from build123d import *

# Parameters (mm, degrees)
F1_DEPTH = 101.6
F3_DEPTH = 6.35
F4_R     = 3.175
F5_DEPTH = 50.801
F6_R     = 6.35
F7_DEPTH = 6.35


with BuildPart() as f1:
    # F0 (on Front) → F1 (new body)
    with BuildSketch(Plane.XZ):
        Polygon((0, 50.8), (0, 0), (148.59, 0), (148.59, 12.7), (135.89, 12.7), (135.89, 25.4), (123.19, 25.4), (123.19, 38.1), (110.49, 38.1), (110.49, 50.8), align=None)
    extrude(amount=F1_DEPTH)

    # F2 (on face) → F3 (cut)
    with BuildSketch(Plane.XY.offset(50.8)):
        with BuildLine():
            ThreePointArc((25.4, -31.75), (29.890128, -29.890128), (31.75, -25.4))
            ThreePointArc((31.75, -25.4), (29.890128, -20.909872), (25.4, -19.05))
            ThreePointArc((25.4, -19.05), (19.05, -25.4), (25.4, -31.75))
        make_face()
        with BuildLine():
            ThreePointArc((25.4, -19.05), (29.890128, -20.909872), (31.75, -25.4))
            ThreePointArc((31.75, -25.4), (29.890128, -29.890128), (25.4, -31.75))
            Line((25.4, -31.75), (101.6, -31.75))
            ThreePointArc((101.6, -31.75), (95.25, -25.4), (101.6, -19.05))
            Line((101.6, -19.05), (25.4, -19.05))
        make_face()
        with BuildLine():
            ThreePointArc((107.95, -25.4), (106.090128, -20.909872), (101.6, -19.05))
            ThreePointArc((101.6, -19.05), (95.25, -25.4), (101.6, -31.75))
            ThreePointArc((101.6, -31.75), (106.090128, -29.890128), (107.95, -25.4))
        make_face()
        with BuildLine():
            ThreePointArc((31.75, -76.2), (29.890128, -80.690128), (25.4, -82.55))
            Line((25.4, -82.55), (101.6, -82.55))
            ThreePointArc((101.6, -82.55), (95.25, -76.2), (101.6, -69.85))
            Line((101.6, -69.85), (25.4, -69.85))
            ThreePointArc((25.4, -69.85), (29.890128, -71.709872), (31.75, -76.2))
        make_face()
        with BuildLine():
            ThreePointArc((25.4, -69.85), (19.05, -76.2), (25.4, -82.55))
            ThreePointArc((25.4, -82.55), (29.890128, -80.690128), (31.75, -76.2))
            ThreePointArc((31.75, -76.2), (29.890128, -71.709872), (25.4, -69.85))
        make_face()
        with BuildLine():
            ThreePointArc((101.6, -69.85), (95.25, -76.2), (101.6, -82.55))
            ThreePointArc((101.6, -82.55), (106.090128, -80.690128), (107.95, -76.2))
            ThreePointArc((107.95, -76.2), (106.090128, -71.709872), (101.6, -69.85))
        make_face()
    extrude(amount=-F3_DEPTH, mode=Mode.SUBTRACT)

    # F4 (on face) → F5 (cut, through all)
    with BuildSketch(Plane.XY.offset(50.8)):
        with Locations((101.6, -50.8)):
            Circle(F4_R)
        with Locations((63.5, -50.8)):
            Circle(F4_R)
        with BuildLine():
            ThreePointArc((25.4, -28.575), (27.645064, -27.645064), (28.575, -25.4))
            ThreePointArc((28.575, -25.4), (27.645064, -23.154936), (25.4, -22.225))
            ThreePointArc((25.4, -22.225), (22.225, -25.4), (25.4, -28.575))
        make_face()
        with BuildLine():
            ThreePointArc((25.4, -22.225), (27.645064, -23.154936), (28.575, -25.4))
            ThreePointArc((28.575, -25.4), (27.645064, -27.645064), (25.4, -28.575))
            Line((25.4, -28.575), (101.6, -28.575))
            ThreePointArc((101.6, -28.575), (98.425, -25.4), (101.6, -22.225))
            Line((101.6, -22.225), (25.4, -22.225))
        make_face()
        with BuildLine():
            ThreePointArc((104.775, -25.4), (103.845064, -23.154936), (101.6, -22.225))
            ThreePointArc((101.6, -22.225), (98.425, -25.4), (101.6, -28.575))
            ThreePointArc((101.6, -28.575), (103.845064, -27.645064), (104.775, -25.4))
        make_face()
        with Locations((25.4, -50.8)):
            Circle(F4_R)
        with BuildLine():
            ThreePointArc((25.4, -79.375), (27.645064, -78.445064), (28.575, -76.2))
            ThreePointArc((28.575, -76.2), (27.645064, -73.954936), (25.4, -73.025))
            ThreePointArc((25.4, -73.025), (22.225, -76.2), (25.4, -79.375))
        make_face()
        with BuildLine():
            ThreePointArc((25.4, -73.025), (27.645064, -73.954936), (28.575, -76.2))
            ThreePointArc((28.575, -76.2), (27.645064, -78.445064), (25.4, -79.375))
            Line((25.4, -79.375), (101.6, -79.375))
            ThreePointArc((101.6, -79.375), (98.425, -76.2), (101.6, -73.025))
            Line((101.6, -73.025), (25.4, -73.025))
        make_face()
        with BuildLine():
            ThreePointArc((104.775, -76.2), (103.845064, -73.954936), (101.6, -73.025))
            ThreePointArc((101.6, -73.025), (98.425, -76.2), (101.6, -79.375))
            ThreePointArc((101.6, -79.375), (103.845064, -78.445064), (104.775, -76.2))
        make_face()
    extrude(amount=-F5_DEPTH, mode=Mode.SUBTRACT)

    # F6 (on face) → F7 (cut)
    with BuildSketch(Plane.XY.offset(50.8)):
        with Locations((101.6, -50.8)):
            Circle(F6_R)
        with Locations((63.5, -50.8)):
            Circle(F6_R)
        with Locations((25.4, -50.8)):
            Circle(F6_R)
    extrude(amount=-F7_DEPTH, mode=Mode.SUBTRACT)


solid = f1.part
Can you work these out from the model? Positions are in its coordinate system, mm. A direction names the side the tool comes from. Round coordinates to 2 decimals unless told otherwise and drop trailing zeros. Loops run counter-clockwise (first coordinate to the right, second up) from the corner with the lowest first, then second, coordinate; pieces in that order, holes last. Notation, with made-up numbers: (-0.75, -5) - (15.25, -5) arc R13 cw to (15.25, 19) - close; hole circle Ø5 at (16, 12). An arc over 180 degrees is marked (long way). Write item = value, one per line. Start each with the question number.
(1) If we section it at C-C (y = -10.5): Please give me the cut outline in (x, z), and give its area (3 significant figures).
(2) For faces 1 (the face through (22.226, -25.33, 22.536)), 2 (the face through (66, -54, 44.45)), 3 (the face through (56, -50, 50.8)), which set-ups out of +Z, -Z, +X, -X, +Y, -Y let a thin tool reach every point of the face, with its end or its side?
(3) If we section it at A-A (x = 63.5): Please give me the cut outline in (y, z) (3 decimals).
(4) If we section it at D-D (z = 27.5): Please give me the cut outline in (x, y) (3 decimals), and give its area (3 significant figures).
(5) If we section it at B-B (y = -50.8): Give the number of separate pieces and of enclosed holes in the cut face, and give its area (3 significant figures).
(6) For P1, Ø4, axis at x = 127.5, y = -60.5, coming from the +Z side; P2, Ø6.5, axis at y = -32.5, z = 34.5, coming from the +X side; P3, Ø4, axis at y = -43.5, z = 18.5, coming from the +X side, each with a flat end and sliding along its axis, tell me the tip position at first contact or that it passes through.
(7) If I drill on probe 1 along Y at (x, z) = (101.6, 47.5); probe 2 along Y at (x, z) = (40, 17.5) (3 decimals), over which ranges is the centre line in solid material (lowest first)? Write a range as [from, to].
(8) If we mould it in two halves opening along Y, with no side actions, what happens to faces 4 (the face through (135.89, -50, 19)), 5 (the face through (63, -28.575, 23)), 6 (the face through (73, 0, 26)), 7 (the face through (27.107, -48.123, 22.536))? For each: released by +Y, released by -Y, zero draft, split by the parting line, or undercut.
Ans:
q1.outline = (0, 0) - (148.59, 0) - (148.59, 12.7) - (135.89, 12.7) - (135.89, 25.4) - (123.19, 25.4) - (123.19, 38.1) - (110.49, 38.1) - (110.49, 50.8) - (0, 50.8) - close
q1.area = 6,580 mm²
q2.face_1 = +Z, -Z
q2.face_2 = +Z
q2.face_3 = +Z, +X, -X, +Y, -Y
q3.outline = (-101.6, 0) - (-79.375, 0) - (-79.375, 44.45) - (-82.55, 44.45) - (-82.55, 50.8) - (-101.6, 50.8) - close; (-73.025, 0) - (-53.975, 0) - (-53.975, 44.45) - (-57.15, 44.45) - (-57.15, 50.8) - (-69.85, 50.8) - (-69.85, 44.45) - (-73.025, 44.45) - close; (-47.625, 0) - (-28.575, 0) - (-28.575, 44.45) - (-31.75, 44.45) - (-31.75, 50.8) - (-44.45, 50.8) - (-44.45, 44.45) - (-47.625, 44.45) - close; (-22.225, 0) - (0, 0) - (0, 50.8) - (-19.05, 50.8) - (-19.05, 44.45) - (-22.225, 44.45) - close
q4.outline = (0, -101.6) - (123.19, -101.6) - (123.19, 0) - (0, 0) - close; hole circle Ø6.35 at (25.4, -50.8); hole (25.4, -79.375) - (101.6, -79.375) arc R3.175 ccw to (101.6, -73.025) - (25.4, -73.025) arc R3.175 ccw to start; hole (25.4, -28.575) - (101.6, -28.575) arc R3.175 ccw to (101.6, -22.225) - (25.4, -22.225) arc R3.175 ccw to start; hole circle Ø6.35 at (63.5, -50.8); hole circle Ø6.35 at (101.6, -50.8)
q4.area = 11,400 mm²
q5.separate_pieces = 4
q5.enclosed_holes = 0
q5.area = 5,490 mm²
q6.P1 = 25.4
q6.P2 = 123.19
q6.P3 = 135.89
q7.probe_1 = [-101.6, -82.55], [-69.85, -57.15], [-44.45, -31.75], [-19.05, 0]
q7.probe_2 = [-101.6, -79.375], [-73.025, -28.575], [-22.225, 0]
q8.face_4 = zero draft
q8.face_5 = undercut
q8.face_6 = released by +Y
q8.face_7 = undercut
